The listing builds one solid part. Answer for the finished solid, in the listing's coordinates (mm). Coordinates: 2 decimals unless noted, no trailing zeros. Write each loop counter-clockwise with the first axis right and the second up, starting at its lowest first coordinate (ties: lowest second). Pieces come first, ordered by that corner, then holes.
from build123d import *

# Parameters (mm, degrees)
SKETCH3_W           = 150
SKETCH3_H           = 150
BOSS_EXTRUDE1_DEPTH = 3
SKETCH4_W           = 80
SKETCH4_H           = 80
CUT_EXTRUDE1_DEPTH  = 3
SKETCH5_W           = 35
SKETCH5_H           = 3
BOSS_EXTRUDE2_DEPTH = 10
SKETCH7_W           = 80
SKETCH7_H           = 3
CUT_EXTRUDE2_DEPTH  = 27.5
SKETCH8_W           = 33.2
SKETCH8_H           = 25
CUT_EXTRUDE3_DEPTH  = 3


with BuildPart() as part:
    # Sketch3 → Boss-Extrude1 (new body)
    with BuildSketch(Plane(origin=(0, 0, 0), x_dir=(1, 0, 0), z_dir=(0, 1, 0))):
        Rectangle(SKETCH3_W, SKETCH3_H)
    extrude(amount=BOSS_EXTRUDE1_DEPTH)

    # Sketch4 → Cut-Extrude1 (cut)
    with BuildSketch(Plane(origin=(0, 3, 0), x_dir=(1, 0, 0), z_dir=(0, 1, 0))):
        with Locations((0, 35)):
            Rectangle(SKETCH4_W, SKETCH4_H)
    extrude(amount=-CUT_EXTRUDE1_DEPTH, mode=Mode.SUBTRACT)

    # Sketch5 → Boss-Extrude2 (add)
    with BuildSketch(Plane(origin=(0, 0, -75), x_dir=(-1, 0, 0), z_dir=(0, 0, -1))):
        with Locations((-57.5, 1.5)):
            Rectangle(SKETCH5_W, SKETCH5_H)
        with Locations((57.5, 1.5)):
            Rectangle(SKETCH5_W, SKETCH5_H)
    extrude(amount=BOSS_EXTRUDE2_DEPTH)

    # Sketch7 → Cut-Extrude2 (cut)
    with BuildSketch(Plane(origin=(0, 0, 5), x_dir=(-1, 0, 0), z_dir=(0, 0, -1))):
        with Locations((0, 1.5)):
            Rectangle(SKETCH7_W, SKETCH7_H)
    extrude(amount=-CUT_EXTRUDE2_DEPTH, mode=Mode.SUBTRACT)

    # Sketch8 → Cut-Extrude3 (cut)
    with BuildSketch(Plane(origin=(0, 3, 0), x_dir=(1, 0, 0), z_dir=(0, 1, 0))):
        with Locations((0, -45)):
            Rectangle(SKETCH8_W, SKETCH8_H)
    extrude(amount=-CUT_EXTRUDE3_DEPTH, mode=Mode.SUBTRACT)


solid = part.part
1. Section D-D on x = 5 is taken. Give the vertices of the cut face in (y, z), then the cut area to 3 significant figures.
Results found:
outline: (0, 57.5) - (3, 57.5) - (3, 75) - (0, 75) - close
area: 52.5 mm2
2. Flat-ended cylindrical pins translate along their axes: P1, Ø1.5, axis at x = -4.5, y = 1, coming from the -Z side; P2, Ø0.9, axis at x = -30.5, y = 1, coming from the -Z side. Find the tip coordinate at first contact, or state that the pin passes through.
Results found:
P1: stops at z = 57.5
P2: stops at z = 32.5
3. Find the intervals of material crossed by L1, parallel to X at y = 1.2, z = 49.5; L2, parallel to X at y = 2.3, z = 4.5; L3, parallel to Z at x = 29, y = 1.15, in increasing order.
Results found:
L1: x = -75 to -16.6, 16.6 to 75
L2: x = -75 to -40, 40 to 75
L3: z = 32.5 to 75
4. Section B-B on y = 1.65 is taken. Give the vertices of the cut face in (x, z), then the cut area to 3 significant figures.
Results found:
outline: (-75, -85) - (-40, -85) - (-40, 32.5) - (-16.6, 32.5) - (-16.6, 57.5) - (16.6, 57.5) - (16.6, 32.5) - (40, 32.5) - (40, -85) - (75, -85) - (75, 75) - (-75, 75) - close
area: 13,800 mm2
5. Section C-C on z = -63.5 is taken. Give the vertices of the cut face in (x, y).
Results found:
outline: (-75, 0) - (-40, 0) - (-40, 3) - (-75, 3) - close; (40, 0) - (75, 0) - (75, 3) - (40, 3) - close
6. Section A-A on z = 55 is taken. Give the vertices of the cut face in (x, y).
Results found:
outline: (-75, 0) - (-16.6, 0) - (-16.6, 3) - (-75, 3) - close; (16.6, 0) - (75, 0) - (75, 3) - (16.6, 3) - close
